```python
from build123d import *

# Parameters (mm, degrees)
F1_DEPTH = 10.25
F2_DEPTH = 4.25
F4_DEPTH = 5
F5_W     = 40.916331174
F5_H     = 1
F6_DEPTH = 5
F7_R     = 4.99999


# Not quite as in the source:
# - a fillet or chamfer is up to 0.001 mm smaller than in the source, because OpenCascade refuses the exact size


with BuildPart() as f1:
    # F0 (on Top) → F1 (new body, symmetric)
    with BuildSketch(Plane.XY):
        Polygon((0, 0), (-40, 0), (-40, -1), (0.916331174, -1), (1.0038198375, 0), align=None)
    extrude(amount=F1_DEPTH, both=True)

    # F0 (on Top) → F2 (join, symmetric)
    with BuildSketch(Plane.XY):
        Polygon((4.3577871374, 49.8097349046), (0, 0), (1.0038198375, 0), (5.3539818355, 49.7225791618), align=None)
    extrude(amount=F2_DEPTH, both=True)

    # F3 (on face) → F4 (join)
    with BuildSketch(Plane(origin=(0.9961946981, -0.0871557427, 0), x_dir=(0.0871557427, 0.9961946981, 0), z_dir=(0.9961946981, -0.0871557427, 0))):
        Polygon((50, -4.25), (50, -3.25), (-0.916331174, -3.25), (-0.916331174, -4.25), (0.0874886635, -4.25), align=None)
        Polygon((-0.916331174, 3.25), (50, 3.25), (50, 4.25), (0.0874886635, 4.25), (-0.916331174, 4.25), align=None)
    extrude(amount=F4_DEPTH)

    # F5 (on face) → F6 (join)
    with BuildSketch(Plane.XZ.offset(1)):
        with Locations((-19.541834413, 9.75)):
            Rectangle(F5_W, F5_H)
        with Locations((-19.541834413, -9.75)):
            Rectangle(F5_W, F5_H)
    extrude(amount=F6_DEPTH)

    # F7 (radius 5 in the source; OpenCascade refuses exactly that, so slightly less here)
    f7_edges = [f1.edges().sort_by_distance(p)[0] for p in [
        (0.960076, -0.5, -4.25),
        (0.960076, -0.5, 4.25),
        (0.50191, 0, 4.25),
        (0.50191, 0, -4.25),
        (0, 0, 0),
    ]]
    fillet(f7_edges, radius=F7_R)


solid = f1.part
```
Input: part model. Units: mm. Frame: model coordinates. A direction names the side the tool comes from. Give positions to 0.01 mm unless a question says otherwise; leave off trailing zeros. Order: outer loops, then holes, each group sorted by start corner. A loop starts at its lowest first (then second) coordinate and runs counter-clockwise, first axis right, second up.
1. Material intervals for L1, parallel to Y at x = -35.5, z = 7.5; L2, parallel to X at y = 10, z = -1.75; L3, parallel to X at y = 20, z = 1, sorted ascending.
Derived:
L1: y = -1 to 0
L2: x = 0.87 to 1.88
L3: x = 1.75 to 2.75
2. Reachability of faces 1 (the flat face through (5, 25, 4.25)), 2 (the flat face through (-20, -3, 9.25)), 3 (the flat face through (-20, -1, 0)), 4 (the flat face through (6, 24, 3.25)), 5 (the flat face through (5, 24, -4.25)) from +Z, -Z, +X, -X, +Y, -Y: full face, straight path, thin tool, end or side. Return the list, or none.
Derived:
face 1: +Z, +X, -X, +Y
face 2: +X, -X, -Y
face 3: -X, -Y
face 4: +X, -Y
face 5: -Z, +X, -X, +Y
3. Section A-A on x = -17. Return the cut outline in (y, z), and give its area (3 significant figures).
Derived:
outline: (-6, -10.25) - (0, -10.25) - (0, 10.25) - (-6, 10.25) - (-6, 9.25) - (-1, 9.25) - (-1, -9.25) - (-6, -9.25) - close
area: 30.5 mm2
4. Pin query (flat end, axial travel): pin 1 (2 mm diameter, centred on x = -3.5, z = 7.5, fed in from +Y); pin 2 (10 mm diameter, centred on x = -13.5, z = -4, fed in from +Y); pin 3 (5 mm diameter, centred on x = 3.5, y = 14.5, fed in from +Z); pin 4 (10 mm diameter, centred on x = -0.5, z = 5.5, fed in from -Y). Return the tip coordinate at first contact, or that it passes through.
Derived:
pin 1: stops at y = 0.43
pin 2: stops at y = 0
pin 3: stops at z = 4.25
pin 4: stops at y = -6
5. Section D-D on z = 6. Return the cut outline in (x, y).
Derived:
outline: (-40, -1) - (0.92, -1) - (2.11, -1.1) - (2.31, 1.2) - (-1.33, 1.2) arc R5 cw to (-4.58, 0) - (-40, 0) - close
6. Section B-B on z = 0.75. Return the cut outline in (x, y), and give its area (3 significant figures).
Derived:
outline: (-40, -1) - (0.92, -1) - (5.35, 49.72) - (4.36, 49.81) - (0.4, 4.56) arc R5 cw to (-4.58, 0) - (-40, 0) - close
area: 95.3 mm2
7. Section C-C on z = -5. Return the cut outline in (x, y), and give its area (3 significant figures).
Derived:
outline: (-40, -1) - (0.92, -1) - (3.27, -1.21) - (3.59, 2.37) - (-0.33, 2.37) arc R5 cw to (-4.58, 0) - (-40, 0) - close
area: 55.6 mm2
8. Mould query, pull axis Z, two halves, no side actions, for faces 6 (the cylindrical face through (3.156, 0.651, -5.186)), 7 (the flat face through (-20, -3, -9.25)), 8 (the flat face through (8.085, 23.57, 3.757)), 9 (the cylindrical face through (1.02, 1.5, 5.68)). Classes: released by +Z, released by -Z, zero draft, split by the parting line, or undercut.
Derived:
face 6: released by -Z
face 7: undercut
face 8: zero draft
face 9: released by +Z
